For this review, take the finished solid that the model builds, in its own axes (mm). A direction names the side the tool comes from. Give positions to 0.01 mm unless a question says otherwise; leave off trailing zeros. Loops run counter-clockwise (first coordinate to the right, second up) from the corner with the lowest first, then second, coordinate; pieces in that order, holes last.
```python
from build123d import *

# Parameters (mm, degrees)
Y_KSEKLIK_EKSTR_ZYON1_DEPTH = 60


with BuildPart() as part:
    # Çizim3 → Yükseklik-Ekstrüzyon1 (new body)
    with BuildSketch(Plane.XY):
        with BuildLine():
            Line((51, 0), (59.481089432, 0))
            ThreePointArc((59.481089432, 0), (60.555036053, 0.452794836), (60.980612695, 1.537815126))
            ThreePointArc((60.980612695, 1.537815126), (56.356651483, 23.343689374), (44.207204261, 42.032405254))
            ThreePointArc((44.207204261, 42.032405254), (43.139050927, 42.498702329), (42.05948169, 42.05948169))
            Line((42.05948169, 42.05948169), (36.062445841, 36.062445841))
            ThreePointArc((36.062445841, 36.062445841), (36.018511858, 35.956379823), (36.062445841, 35.850313806))
            Line((36.062445841, 35.850313806), (36.203867197, 35.70889245))
            ThreePointArc((36.203867197, 35.70889245), (36.24780118, 35.602826433), (36.203867197, 35.496760416))
            Line((36.203867197, 35.496760416), (35.885669145, 35.178562364))
            ThreePointArc((35.885669145, 35.178562364), (35.841735162, 35.072496347), (35.885669145, 34.96643033))
            Line((35.885669145, 34.96643033), (36.875618639, 33.976480836))
            ThreePointArc((36.875618639, 33.976480836), (36.981684656, 33.932546853), (37.087750673, 33.976480836))
            Line((37.087750673, 33.976480836), (39.636467242, 36.525197405))
            ThreePointArc((39.636467242, 36.525197405), (40.022243815, 36.684991294), (40.408020388, 36.525197405))
            Line((40.408020388, 36.525197405), (42.112435937, 34.820781856))
            ThreePointArc((42.112435937, 34.820781856), (42.239327901, 34.621601371), (42.270153765, 34.387455685))
            Line((42.270153765, 34.387455685), (41.822915851, 29.275502936))
            ThreePointArc((41.822915851, 29.275502936), (41.773876207, 29.092484494), (41.665198023, 28.937275961))
            Line((41.665198023, 28.937275961), (36.116547908, 23.388625846))
            ThreePointArc((36.116547908, 23.388625846), (35.961339375, 23.279947662), (35.778320934, 23.230908018))
            Line((35.778320934, 23.230908018), (30.666368185, 22.783670104))
            ThreePointArc((30.666368185, 22.783670104), (30.432222498, 22.814495969), (30.233042013, 22.941387932))
            Line((30.233042013, 22.941387932), (28.528626464, 24.645803481))
            ThreePointArc((28.528626464, 24.645803481), (28.368832576, 25.031580054), (28.528626464, 25.417356627))
            Line((28.528626464, 25.417356627), (31.077343033, 27.966073196))
            ThreePointArc((31.077343033, 27.966073196), (31.121277016, 28.072139213), (31.077343033, 28.17820523))
            Line((31.077343033, 28.17820523), (30.087393539, 29.168154724))
            ThreePointArc((30.087393539, 29.168154724), (29.981327522, 29.212088707), (29.875261505, 29.168154724))
            Line((29.875261505, 29.168154724), (29.557063454, 28.849956672))
            ThreePointArc((29.557063454, 28.849956672), (29.450997436, 28.80602269), (29.344931419, 28.849956672))
            Line((29.344931419, 28.849956672), (29.203510063, 28.991378029))
            ThreePointArc((29.203510063, 28.991378029), (29.097444046, 29.035312011), (28.991378029, 28.991378029))
            Line((28.991378029, 28.991378029), (22.956480566, 22.956480566))
            ThreePointArc((22.956480566, 22.956480566), (22.517540413, 21.930445005), (22.90865732, 20.885244069))
            ThreePointArc((22.90865732, 20.885244069), (28.640265508, 11.863186403), (30.966964646, 1.430769231))
            ThreePointArc((30.966964646, 1.430769231), (31.429471899, 0.415139144), (32.465366161, 0))
            Line((32.465366161, 0), (41, 0))
            ThreePointArc((41, 0), (41.106066017, 0.043933983), (41.15, 0.15))
            Line((41.15, 0.15), (41.15, 0.35))
            ThreePointArc((41.15, 0.35), (41.193933983, 0.456066017), (41.3, 0.5))
            Line((41.3, 0.5), (41.75, 0.5))
            ThreePointArc((41.75, 0.5), (41.856066017, 0.543933983), (41.9, 0.65))
            Line((41.9, 0.65), (41.9, 2.05))
            ThreePointArc((41.9, 2.05), (41.856066017, 2.156066017), (41.75, 2.2))
            Line((41.75, 2.2), (38.145570461, 2.2))
            ThreePointArc((38.145570461, 2.2), (37.759793889, 2.359793889), (37.6, 2.745570461))
            Line((37.6, 2.745570461), (37.6, 5.155978046))
            ThreePointArc((37.6, 5.155978046), (37.651115704, 5.386546086), (37.794884529, 5.573909267))
            Line((37.794884529, 5.573909267), (41.725825944, 8.872360759))
            ThreePointArc((41.725825944, 8.872360759), (41.88991579, 8.967098075), (42.076511877, 9))
            Line((42.076511877, 9), (49.923488123, 9))
            ThreePointArc((49.923488123, 9), (50.11008421, 8.967098075), (50.274174056, 8.872360759))
            Line((50.274174056, 8.872360759), (54.205115471, 5.573909267))
            ThreePointArc((54.205115471, 5.573909267), (54.348884296, 5.386546086), (54.4, 5.155978046))
            Line((54.4, 5.155978046), (54.4, 2.745570461))
            ThreePointArc((54.4, 2.745570461), (54.240206111, 2.359793889), (53.854429539, 2.2))
            Line((53.854429539, 2.2), (50.25, 2.2))
            ThreePointArc((50.25, 2.2), (50.143933983, 2.156066017), (50.1, 2.05))
            Line((50.1, 2.05), (50.1, 0.65))
            ThreePointArc((50.1, 0.65), (50.143933983, 0.543933983), (50.25, 0.5))
            Line((50.25, 0.5), (50.7, 0.5))
            ThreePointArc((50.7, 0.5), (50.806066017, 0.456066017), (50.85, 0.35))
            Line((50.85, 0.35), (50.85, 0.15))
            ThreePointArc((50.85, 0.15), (50.893933983, 0.043933983), (51, 0))
        make_face()
        with BuildLine():
            Line((56.945570461, 2.2), (58.389915016, 2.2))
            ThreePointArc((58.389915016, 2.2), (58.784647482, 2.368962697), (58.934883346, 2.771195588))
            ThreePointArc((58.934883346, 2.771195588), (54.508892418, 22.57832251), (43.632786855, 39.71372447))
            ThreePointArc((43.632786855, 39.71372447), (43.242132452, 39.891913277), (42.843539779, 39.732269942))
            Line((42.843539779, 39.732269942), (41.82223395, 38.710964113))
            ThreePointArc((41.82223395, 38.710964113), (41.662440062, 38.32518754), (41.82223395, 37.939410967))
            Line((41.82223395, 37.939410967), (44.186108114, 35.575536804))
            ThreePointArc((44.186108114, 35.575536804), (44.313000077, 35.376356319), (44.343825942, 35.142210633))
            Line((44.343825942, 35.142210633), (43.751861055, 28.376021015))
            ThreePointArc((43.751861055, 28.376021015), (43.702821411, 28.193002574), (43.594143227, 28.037794041))
            Line((43.594143227, 28.037794041), (39.029162165, 23.472812979))
            ThreePointArc((39.029162165, 23.472812979), (38.869368276, 23.087036406), (39.029162165, 22.701259833))
            Line((39.029162165, 22.701259833), (39.209750843, 22.520671155))
            ThreePointArc((39.209750843, 22.520671155), (39.518169578, 22.366389496), (39.857496647, 22.42788817))
            ThreePointArc((39.857496647, 22.42788817), (47.579795924, 19.708196767), (44.042417973, 12.324594348))
            ThreePointArc((44.042417973, 12.324594348), (43.758991372, 12.128140006), (43.65, 11.800961419))
            Line((43.65, 11.800961419), (43.65, 11.545570461))
            ThreePointArc((43.65, 11.545570461), (43.809793889, 11.159793889), (44.195570461, 11))
            Line((44.195570461, 11), (50.651428591, 11))
            ThreePointArc((50.651428591, 11), (50.838024679, 10.967098075), (51.002114524, 10.872360759))
            Line((51.002114524, 10.872360759), (56.205115471, 6.506524583))
            ThreePointArc((56.205115471, 6.506524583), (56.348884296, 6.319161403), (56.4, 6.088593363))
            Line((56.4, 6.088593363), (56.4, 2.745570461))
            ThreePointArc((56.4, 2.745570461), (56.559793889, 2.359793889), (56.945570461, 2.2))
        make_face(mode=Mode.SUBTRACT)
        with BuildLine():
            Line((35.054429539, 2.2), (32.931315946, 2.2))
            ThreePointArc((32.931315946, 2.2), (32.561912844, 2.344087614), (32.387631786, 2.700242082))
            ThreePointArc((32.387631786, 2.700242082), (30.026084807, 12.437211552), (24.81087355, 20.992154575))
            ThreePointArc((24.81087355, 20.992154575), (24.682269628, 21.367229133), (24.841591738, 21.730321901))
            Line((24.841591738, 21.730321901), (26.342859756, 23.231589919))
            ThreePointArc((26.342859756, 23.231589919), (26.728636329, 23.391383807), (27.114412902, 23.231589919))
            Line((27.114412902, 23.231589919), (29.478287065, 20.867715756))
            ThreePointArc((29.478287065, 20.867715756), (29.67746755, 20.740823792), (29.911613237, 20.709997927))
            Line((29.911613237, 20.709997927), (36.622183037, 21.297096711))
            ThreePointArc((36.622183037, 21.297096711), (36.856328724, 21.266270846), (37.055509209, 21.139378882))
            Line((37.055509209, 21.139378882), (37.485300638, 20.709587454))
            ThreePointArc((37.485300638, 20.709587454), (37.638184329, 20.410368657), (37.586740146, 20.07831624))
            ThreePointArc((37.586740146, 20.07831624), (37.417121067, 15.498679011), (40.775352408, 12.380325272))
            ThreePointArc((40.775352408, 12.380325272), (41.046525454, 12.181905286), (41.15, 11.862220551))
            Line((41.15, 11.862220551), (41.15, 11.254403684))
            ThreePointArc((41.15, 11.254403684), (41.098884296, 11.023835644), (40.955115471, 10.836472464))
            Line((40.955115471, 10.836472464), (35.794884529, 6.506524583))
            ThreePointArc((35.794884529, 6.506524583), (35.651115704, 6.319161403), (35.6, 6.088593363))
            Line((35.6, 6.088593363), (35.6, 2.745570461))
            ThreePointArc((35.6, 2.745570461), (35.440206111, 2.359793889), (35.054429539, 2.2))
        make_face(mode=Mode.SUBTRACT)
        with BuildLine():
            Line((45.161707445, 19.874363918), (45.645032532, 20.153411787))
            ThreePointArc((45.645032532, 20.153411787), (46.512534009, 19.920965467), (46.280087689, 19.05346399))
            Line((46.280087689, 19.05346399), (45.796762602, 18.774416121))
            ThreePointArc((45.796762602, 18.774416121), (45.529547409, 15.853437889), (43.133513652, 14.161533627))
            Line((43.133513652, 14.161533627), (43.133513652, 13.603437889))
            ThreePointArc((43.133513652, 13.603437889), (42.498458496, 12.968382732), (41.863403339, 13.603437889))
            Line((41.863403339, 13.603437889), (41.863403339, 14.161533627))
            ThreePointArc((41.863403339, 14.161533627), (39.467369582, 15.853437889), (39.200154389, 18.774416121))
            Line((39.200154389, 18.774416121), (38.716829302, 19.05346399))
            ThreePointArc((38.716829302, 19.05346399), (38.484382982, 19.920965467), (39.351884459, 20.153411787))
            Line((39.351884459, 20.153411787), (39.835209546, 19.874363918))
            ThreePointArc((39.835209546, 19.874363918), (42.498458496, 21.103437889), (45.161707445, 19.874363918))
        make_face(mode=Mode.SUBTRACT)
    extrude(amount=-Y_KSEKLIK_EKSTR_ZYON1_DEPTH)


solid = part.part
```
Item 1: Take a section at A-A on x = 34. Give the boundary of the cut face in (y, z), and give its area (3 significant figures).
Answer:
outline: (0, -60) - (2.2, -60) - (2.2, 0) - (0, 0) - close; (21.07, -60) - (23.08, -60) - (23.08, 0) - (21.07, 0) - close
area: 252 mm2
Item 2: The part is to be moulded in two halves that separate along X. For faces 1 (the cylindrical face through (56.476, 23.053, -29.58)), 2 (the cylindrical face through (30.08, 12.31, -29.58)), 3 (the flat face through (26, 26, -30)), say which applies: released by +X, released by -X, zero draft, split by the parting line, or undercut.
Answer:
face 1: released by +X
face 2: undercut
face 3: released by -X
Item 3: Take a section at D-D on z = -37. State how many separate pieces and enclosed holes the cut face has, and give its area (3 significant figures).
Answer:
separate pieces: 1
enclosed holes: 3
area: 385 mm2
Item 4: Take a section at B-B on y = 33. Give the boundary of the cut face in (x, z), and give its area (3 significant figures).
Answer:
outline: (42.15, -60) - (44.16, -60) - (44.16, 0) - (42.15, 0) - close; (48.91, -60) - (51.3, -60) - (51.3, 0) - (48.91, 0) - close
area: 264 mm2
Item 5: Tool access review of faces 4 (the cylindrical face through (42.51, 12.97, -29.58)), 5 (the flat face through (46, 9, -30)): name each direction out of +Z, -Z, +X, -X, +Y, -Y from which nothing blocks a thin tool from reaching the whole face with its end or side.
Answer:
face 4: +Z, -Z
face 5: +Z, -Z, -Y
Item 6: For L1, parallel to X at y = 6, z = -37.5; L2, parallel to Y at x = 45.5, z = -40; L3, parallel to X at y = 36, z = -19 (3 decimals), list the stretches that pass through material, from the lowest coordinate up.
Answer:
L1: x = 30.41 to 31.94, 35.6 to 38.3, 53.7 to 56.4, 58.69 to 60.7
L2: y = 9 to 11, 12.99 to 15.8, 20.07 to 22.21, 37.56 to 40.63
L3: x = 36.025 to 39.111, 40.933 to 43.762, 46.744 to 49.244
Item 7: Take a section at C-C on y = 10. Give the boundary of the cut face in (x, z).
Answer:
outline: (29.34, -60) - (30.92, -60) - (30.92, 0) - (29.34, 0) - close; (39.96, -60) - (52.04, -60) - (52.04, 0) - (39.96, 0) - close; (58.15, -60) - (60.17, -60) - (60.17, 0) - (58.15, 0) - close
Item 8: Clearance check with flat-ended pins moving along their axes: pin 1 Ø0.7 at (y, z) = (1, -40.5) entering from -X; pin 2 Ø5 at (y, z) = (33, -7) entering from -X; pin 3 Ø4 at (x, z) = (46, -42.5) entering from -Y. State where each tip first meets the part, or that it passes through.
Answer:
pin 1: stops at x = 30.97
pin 2: stops at x = 35.84
pin 3: stops at y = 9
